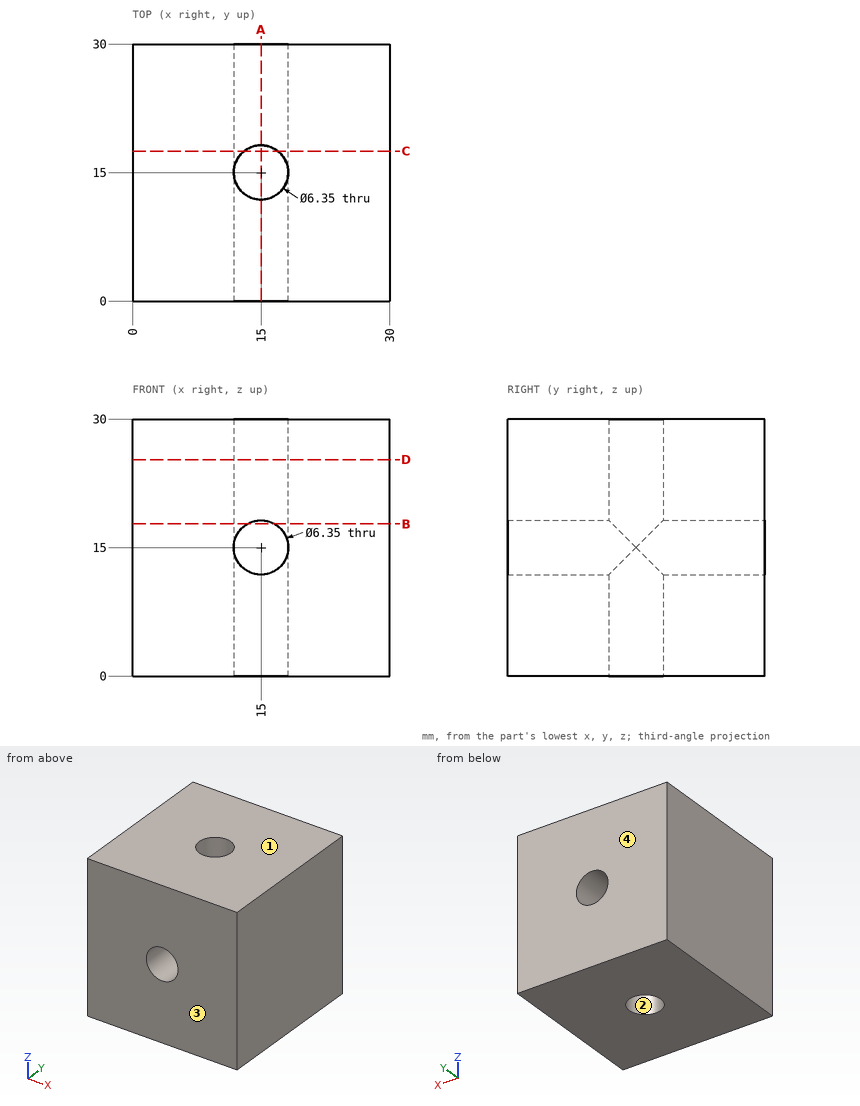
Here's the drawing with two shaded views (mm, measured from the low corner). I have some questions. Coordinates: 2 decimals unless noted, no trailing zeros. Order: outer loops, then holes, each group sorted by start corner. A loop starts at its lowest first (then second) coordinate and runs counter-clockwise, first axis right, second up. Notation, with made-up numbers: (35.25, 37.5) - (40.25, 37.5) arc R12 ccw to (40.25, 54.5) - close; hole circle Ø4 at (-24, -23). An arc over 180 degrees is marked (long way). Answer in a Markdown table with one row per item. Add a question column.
(1) If we section it at C-C, the plane y = 17.5: Please give me the cut outline in (x, z) (3 decimals), then the cut area to 3 significant figures.
(2) If we section it at A-A, the plane x = 15: Please give me the cut outline in (y, z) (3 decimals), then the cut area to 3 significant figures.
(3) I need wall thicknesses on L1, parallel to Z at x = 15, y = 23.75 (3 decimals). Which ranges of the line are inside material? Lowest first, please.
(4) If we mould it in two halves opening along Y, with no side actions, what happens to the marked faces 1, 2, 3 and 4? For each: released by +Y, released by -Y, zero draft, split by the parting line, or undercut.
(5) If we section it at D-D, the plane z = 25.25: Please give me the cut outline in (x, y) (3 decimals), then the cut area to 3 significant figures.
(6) If we section it at B-B, the plane z = 17.75: Please give me the cut outline in (x, y) (3 decimals), then the cut area to 3 significant figures.
Results are:
| question | item | result |
|---|---|---|
| 1 | outline | (0, 0) - (13.043, 0) - (13.043, 12.5) arc R3.175 cw to (13.043, 17.5) - (13.043, 30) - (0, 30) - close; (16.957, 0) - (30, 0) - (30, 30) - (16.957, 30) - (16.957, 17.5) arc R3.175 cw to (16.957, 12.5) - close |
| 1 | area | 774 mm2 |
| 2 | outline | (0, 0) - (11.825, 0) - (11.825, 11.825) - (0, 11.825) - close; (0, 18.175) - (11.825, 18.175) - (11.825, 30) - (0, 30) - close; (18.175, 0) - (30, 0) - (30, 11.825) - (18.175, 11.825) - close; (18.175, 18.175) - (30, 18.175) - (30, 30) - (18.175, 30) - close |
| 2 | area | 559 mm2 |
| 3 | L1 | z = 0 to 11.825, 18.175 to 30 |
| 4 | face 1 | zero draft |
| 4 | face 2 | undercut |
| 4 | face 3 | released by -Y |
| 4 | face 4 | released by +Y |
| 5 | outline | (0, 0) - (30, 0) - (30, 30) - (0, 30) - close; hole circle Ø6.35 at (15, 15) |
| 5 | area | 868 mm2 |
| 6 | outline | (0, 0) - (13.413, 0) - (13.413, 12.25) arc R3.175 cw to (13.413, 17.75) - (13.413, 30) - (0, 30) - close; (16.587, 0) - (30, 0) - (30, 30) - (16.587, 30) - (16.587, 17.75) arc R3.175 cw to (16.587, 12.25) - close |
| 6 | area | 792 mm2 |
